Geometry: final body of the model. Coordinates: model frame, mm. Give positions to 0.01 mm unless a question says otherwise; leave off trailing zeros. Write each loop counter-clockwise with the first axis right and the second up, starting at its lowest first coordinate (ties: lowest second). Pieces come first, ordered by that corner, then holes. Notation, with made-up numbers: M 74,-38.5 L 78,-38.5 A27 ccw 78,-19.5 Z; hole C 40,58 d5. An arc over 180 degrees is marked long. Use a Markdown table: item, result. Add a question column.
1) Line query: line 1 (X direction, y = 52, z = 1.75); line 2 (X direction, y = 8, z = 3.5); line 3 (Y direction, x = -8, z = 19.75). Output: solid intervals per line, ascending.
2) Pin query (flat end, axial travel): pin 1 (5 mm diameter, centred on y = 188, z = 21, fed in from -X). Return the tip coordinate at first contact, or that it passes through.
3) Section A-A on z = 11.5. Return the cut outline in (x, y), then the cut area to 3 significant figures.
4) Section B-B on y = -200. Return the cut outline in (x, z), then the cut area to 3 significant figures.
5) Section C-C on x = -174. Return the cut outline in (y, z), then the cut area to 3 significant figures.
```python
from build123d import *

# Parameters (mm, degrees)
BOSS_EXTRUDE1_DEPTH = 30
FILLET1_R           = 10
FILLET2_R           = 10


with BuildPart() as part:
    # Sketch1 → Boss-Extrude1 (new body)
    with BuildSketch(Plane.XY):
        Polygon((0, 0), (0, 299.049703647), (-191.735, 299.049703647), (-168.625, -246.950296353), (0, -246.950296353), align=None)
    extrude(amount=BOSS_EXTRUDE1_DEPTH)

    # Fillet1
    fillet1_edges = [part.edges().sort_by_distance(p)[0] for p in [
        (-191.735, 299.049703647, 15),
        (0, 299.049703647, 15),
    ]]
    fillet(fillet1_edges, radius=FILLET1_R)

    # Fillet2
    fillet2_edges = [part.edges().sort_by_distance(p)[0] for p in [
        (0, -246.950296353, 15),
        (-168.625, -246.950296353, 15),
    ]]
    fillet(fillet2_edges, radius=FILLET2_R)


solid = part.part
```
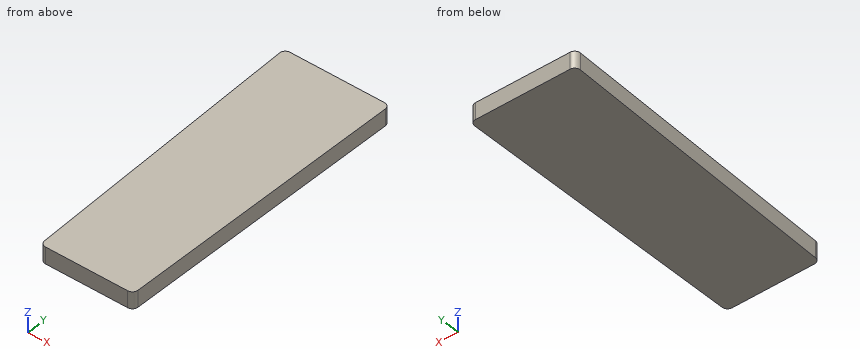
Found:
| question | item | result |
|---|---|---|
| 1 | line 1 | -181.28 to 0 |
| 1 | line 2 | -179.42 to 0 |
| 1 | line 3 | -246.75 to 298.85 |
| 2 | pin 1 | x = -187.14 |
| 3 | outline | M -191.29,288.63 L -169.03,-237.37 A10 ccw -159.04,-246.95 L -10,-246.95 A10 ccw 0,-236.95 L 0,289.05 A10 ccw -10,299.05 L -181.3,299.05 A10 ccw Z |
| 3 | area | 98,300 mm² |
| 4 | outline | M -170.61,0 L 0,0 L 0,30 L -170.61,30 Z |
| 4 | area | 5,120 mm² |
| 5 | outline | M -119.96,0 L 299.05,0 L 299.05,30 L -119.96,30 Z |
| 5 | area | 12,600 mm² |
